Could you check a few things on this drawing? It's one solid part, dimensions in mm from its lowest x, y, z. Round coordinates to 2 decimals unless told otherwise and drop trailing zeros. Loops run counter-clockwise (first coordinate to the right, second up) from the corner with the lowest first, then second, coordinate; pieces in that order, holes last. Notation, with made-up numbers: (75, 9) -> (117, 9) arc R18 cw to (117, 44) -> close; hole circle Ø10 at (69, 76.25). An arc over 180 degrees is marked (long way). Use one line per item in the form item = value. Start each with the question number.
Item 1: Thinking about a two-plate mould opening in Z: for the marked faces 1 and 2, which applies, released by +Z, released by -Z, zero draft, split by the parting line, or undercut?
Item 2: If we section it at A-A (x = 169): Write out the boundary of the cut face in (y, z).
Item 3: If we section it at D-D (z = 240): Write out the boundary of the cut face in (x, y).
Item 4: If I drill on L1, parallel to Z at x = 176, y = 19.5; L2, parallel to Z at x = 144.5, y = 17.75 (1 decimal); L3, parallel to Z at x = 146, y = 11.5, over which ranges is the centre line in solid material (lowest first)? Write a range as [from, to].
Item 5: I'm going to push flat-ended pins straight in: pin 1 Ø7.5 at (x, y) = (141, 18) entering from +Z; pin 2 Ø4 at (y, z) = (14.5, 337) entering from +X; pin 3 Ø5 at (y, z) = (8.5, 108.5) entering from -X. Where does each tip first touch, or does it pass through?
Item 6: If we section it at C-C (x = 124.5): State how many separate pieces and enclosed holes the cut face has, then the cut area to 3 significant figures.
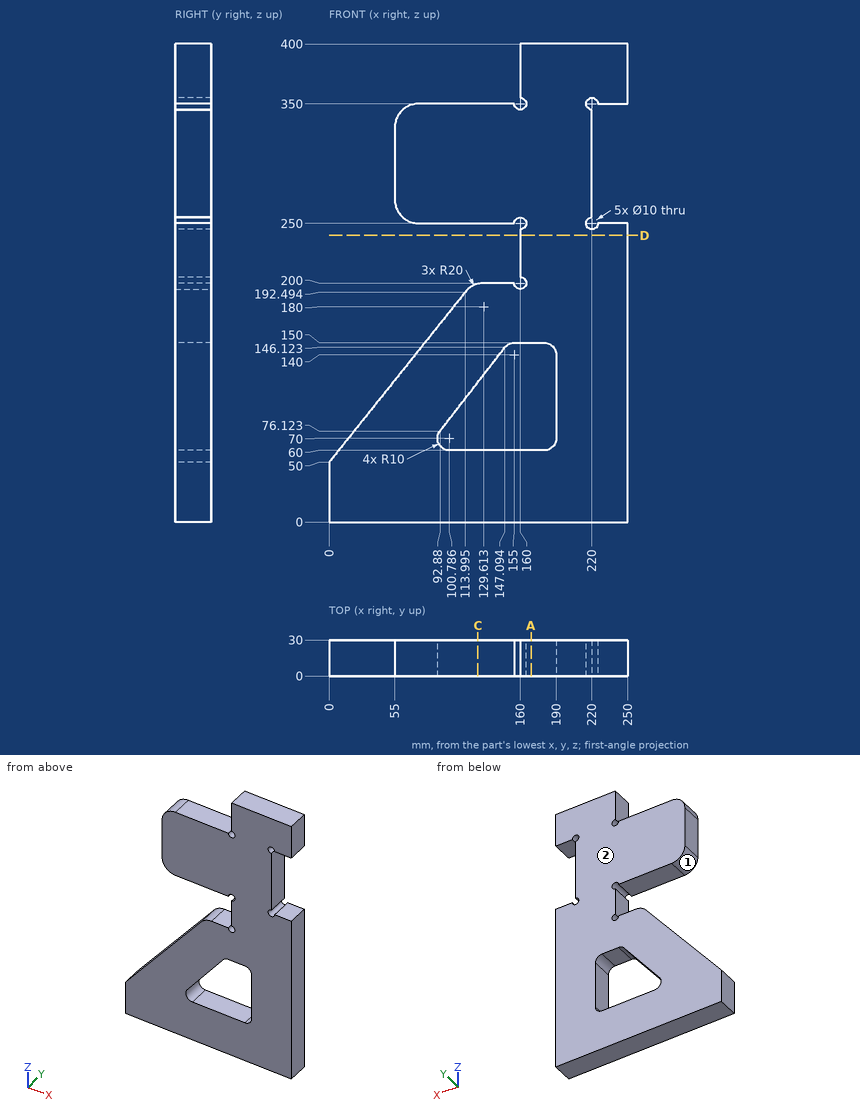
Values found:
q1.face_1 = undercut
q1.face_2 = zero draft
q2.outline = (0, 0) -> (30, 0) -> (30, 60) -> (0, 60) -> close; (0, 150) -> (30, 150) -> (30, 400) -> (0, 400) -> close
q3.outline = (160, 0) -> (250, 0) -> (250, 30) -> (160, 30) -> close
q4.L1 = [0, 60], [150, 400]
q4.L2 = [0, 60], [142.8, 200], [250, 350]
q4.L3 = [0, 60], [144.71, 200], [250, 350]
q5.pin_1 = 350
q5.pin_2 = 220
q5.pin_3 = 44.8
q6.separate_pieces = 3
q6.enclosed_holes = 0
q6.area = 7,270 mm2
